Print and shaded views of the part. All mm, measured from the part's lowest x, y and z. Coordinates: 2 decimals unless noted, no trailing zeros. Loops run counter-clockwise (first coordinate to the right, second up) from the corner with the lowest first, then second, coordinate; pieces in that order, holes last. Notation, with made-up numbers: (77, 5.5) -> (85, 5.5) arc R15 cw to (85, 30.5) -> close; hole circle Ø11 at (30.25, 0.25). An arc over 180 degrees is marked (long way). One line per item, written item: value. Start each with the question number.
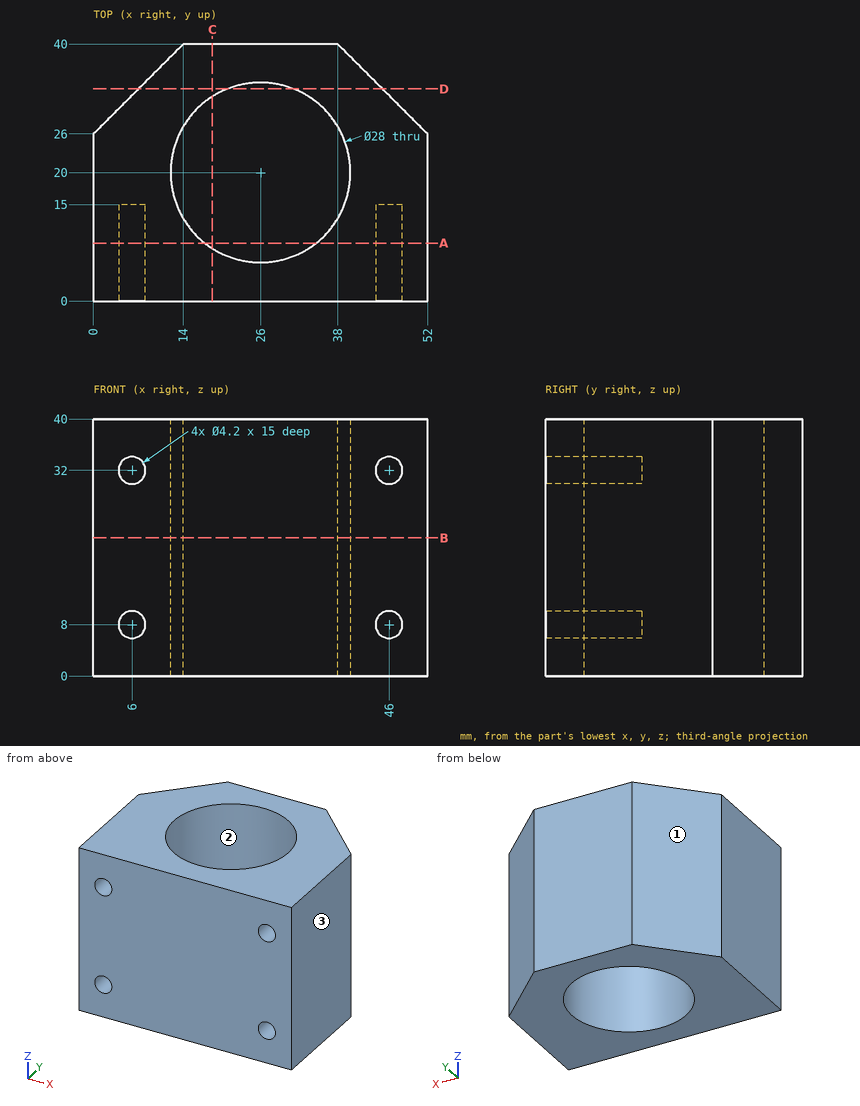
1) Slice it at D-D (y = 33). Give the cut face in (x, z), then the cut area to 3 significant figures.
2) Slice it at B-B (z = 21.5). Give the cut face in (x, y), then the cut area to 3 significant figures.
3) Probe line 1 (Z direction, x = 46, y = 9); line 2 (Y direction, x = 23.5, z = 33); line 3 (Y direction, x = 36, z = 35). List the from-to ranges inside material, lowest first. Write a range as from..to.
4) Pull direction Y, two halves, no side cores. Call the marked faces 1, 2 and 3: +Y half, -Y half, draft (parallel to the pull), parting line (faces both ways), or undercut.
5) Pin check, flat tips, straight feed: pin 1 Ø5 at (x, z) = (46, 8) entering from +Y; pin 2 Ø3.5 at (x, z) = (6, 8) entering from +Y; pin 3 Ø2 at (x, z) = (11, 27) entering from +Y. Stop position of each tip, or through.
6) Slice it at A-A (y = 9). Give the cut face in (x, z), then the cut area to 3 significant figures.
7) Slice it at C-C (x = 18.5). Give the cut face in (y, z).
Check sheet entries:
1. outline: (7, 0) -> (20.8, 0) -> (20.8, 40) -> (7, 40) -> close; (31.2, 0) -> (45, 0) -> (45, 40) -> (31.2, 40) -> close
1. area: 1,100 mm^2
2. outline: (0, 0) -> (52, 0) -> (52, 26) -> (38, 40) -> (14, 40) -> (0, 26) -> close; hole circle Ø28 at (26, 20)
2. area: 1,270 mm^2
3. line 1: z = 0..5.9, 10.1..29.9, 34.1..40
3. line 2: y = 0..6.23, 33.77..40
3. line 3: y = 0..10.2, 29.8..40
4. face 1: +Y half
4. face 2: undercut
4. face 3: draft
5. pin 1: stops at y = 34.5
5. pin 2: stops at y = 33.75
5. pin 3: stops at y = 38
6. outline: (0, 0) -> (17.34, 0) -> (17.34, 40) -> (0, 40) -> close; (34.66, 0) -> (52, 0) -> (52, 40) -> (34.66, 40) -> close; hole circle Ø4.2 at (6, 8); hole circle Ø4.2 at (6, 32); hole circle Ø4.2 at (46, 8); hole circle Ø4.2 at (46, 32)
6. area: 1,330 mm^2
7. outline: (0, 0) -> (8.18, 0) -> (8.18, 40) -> (0, 40) -> close; (31.82, 0) -> (40, 0) -> (40, 40) -> (31.82, 40) -> close
